from build123d import *

# Parameters (mm, degrees)
F0_R     = 4.5
F1_DEPTH = 5
F2_DEPTH = 3.3
F3_R     = 5.5
F4_DEPTH = 1
F6_R     = 1.75
F7_DEPTH = 10


# Not quite as in the source:
# - a fillet or chamfer that OpenCascade refuses, or shapes differently, is made with other operations: its cross-section is extruded or revolved along the edge and cut away or added


with BuildPart() as f1:
    # F0 (on Front) → F1 (new body)
    with BuildSketch(Plane.XZ):
        Circle(F0_R)
    extrude(amount=F1_DEPTH)

    # F2 (add): a face of the model
    f2_faces = [f1.faces().sort_by_distance(p)[0] for p in [
        (0, 0, 0),
    ]]
    extrude(f2_faces, amount=F2_DEPTH)

    # F3 (on Front) → F4 (join)
    with BuildSketch(Plane.XZ):
        Circle(F3_R)
    extrude(amount=F4_DEPTH)

    # F5: fillet of radius 5 on 1 edges, made by hand

    # F5_s1 → F5_t2 (revolve)
    with BuildSketch(Plane.XY):
        with BuildLine():
            ThreePointArc((5.5, -1), (4.7565835097, -2.4188611699), (4.5, -4))
            Line((4.5, -4), (4.5, -1))
            Line((4.5, -1), (5.5, -1))
        make_face()
    revolve(axis=Axis((0, -1, 0), (0, 1, 0)))

    # F6 (on face) → F7 (join)
    with BuildSketch(Plane(origin=(0, 3.3, 0), x_dir=(-1, 0, 0), z_dir=(0, 1, 0))):
        Circle(F6_R)
    extrude(amount=F7_DEPTH)


solid = f1.part
Part model, mm, in its own coordinate system. A direction names the side the tool comes from. Give positions to 0.01 mm unless a question says otherwise; leave off trailing zeros. Order: outer loops, then holes, each group sorted by start corner. A loop starts at its lowest first (then second) coordinate and runs counter-clockwise, first axis right, second up. Notation, with made-up numbers: (11.25, -24) - (20.25, -24) arc R23 ccw to (20.25, 14) - close; hole circle Ø7 at (89, 63.5). An arc over 180 degrees is marked (long way). Use a Markdown table: item, result.
1) Saw through at D-D on y = 0.25. List the corners of the cut face in (x, z), plus the area to 3 significant figures.
Checked values:
| item | result |
|---|---|
| outline | circle Ø9 at (0, 0) |
| area | 63.6 mm² |
2) Flat gauge pins, fed straight in: P1, Ø1.5, axis at y = -1.5, z = -3, coming from the +X side; P2, Ø6, axis at x = 0.5, y = -0.5, coming from the -Z side; P3, Ø1, axis at x = 3.5, y = 2.5, coming from the -Z side; P4, Ø6, axis at x = 1, y = 3.5, coming from the +Z side. Where does each tip first touch, or does it go through?
Checked values:
| item | result |
|---|---|
| P1 | x = 4.93 |
| P2 | z = -5.5 |
| P3 | z = -3.35 |
| P4 | z = 4.5 |
3) 3-axis set-ups, long thin cutter, end or side, ignore diameter. For faces 1 (the cylindrical face through (-1.19, -0.49, -5.37)), 2 (the flat face through (-5, 0, 0)), 3 (the cylindrical face through (-0.59, -4.51, 4.46)): which of +Z, -Z, +X, -X, +Y, -Y reach the whole face in a straight line?
Checked values:
| item | result |
|---|---|
| face 1 | +Y, -Y |
| face 2 | +Y |
| face 3 | -Y |
4) Saw through at C-C on y = 7.25. List the corners of the cut face in (x, z).
Checked values:
| item | result |
|---|---|
| outline | circle Ø3.5 at (0, 0) |
5) Probe L1, parallel to Y at x = -2.5, z = 1.25; L2, parallel to Y at x = -4.5, z = -3; L3, parallel to X at y = 1.25, z = 1.5. List the from-to ranges inside material, lowest first. Write a range as from..to.
Checked values:
| item | result |
|---|---|
| L1 | -5..3.3 |
| L2 | -1.13..0 |
| L3 | -4.24..4.24 |
6) Saw through at B-B on x = 0. List the corners of the cut face in (y, z).
Checked values:
| item | result |
|---|---|
| outline | (-5, -4.5) - (-4, -4.5) arc R5 cw to (-1, -5.5) - (0, -5.5) - (0, -4.5) - (3.3, -4.5) - (3.3, -1.75) - (13.3, -1.75) - (13.3, 1.75) - (3.3, 1.75) - (3.3, 4.5) - (0, 4.5) - (0, 5.5) - (-1, 5.5) arc R5 cw to (-4, 4.5) - (-5, 4.5) - close |
7) Saw through at A-A on z = 0. List the corners of the cut face in (x, y), plus the area to 3 significant figures.
Checked values:
| item | result |
|---|---|
| outline | (-5.5, -1) arc R5 cw to (-4.5, -4) - (-4.5, -5) - (4.5, -5) - (4.5, -4) arc R5 cw to (5.5, -1) - (5.5, 0) - (4.5, 0) - (4.5, 3.3) - (1.75, 3.3) - (1.75, 13.3) - (-1.75, 13.3) - (-1.75, 3.3) - (-4.5, 3.3) - (-4.5, 0) - (-5.5, 0) - close |
| area | 114 mm² |
